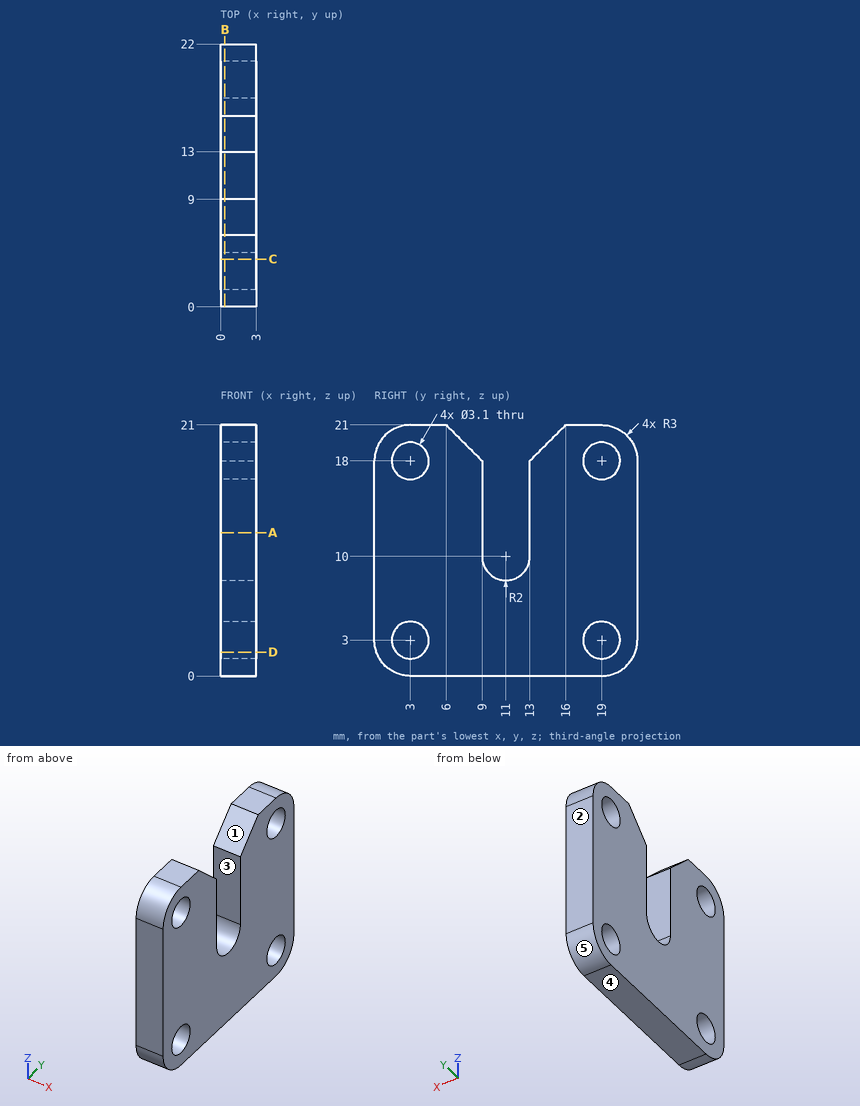
Here's the drawing with two shaded views (mm, measured from the low corner). I have some questions. A direction names the side the tool comes from. Round coordinates to 2 decimals unless told otherwise and drop trailing zeros. Loops run counter-clockwise (first coordinate to the right, second up) from the corner with the lowest first, then second, coordinate; pieces in that order, holes last.
Item 1: Suppose I cut it at B-B, the plane x = 0.35. Write out the boundary of the cut face in (y, z), then the cut area to 3 significant figures.
Item 2: Please list where these lines run through material, in increasing order: L1, parallel to Y at x = 2.1, z = 3; L2, parallel to Y at x = 0.95, z = 12.25; L3, parallel to Y at x = 1, z = 17.25.
Item 3: Will these pins go through, and if not, where does the flat tip stop? pin 1 Ø1.5 at (x, z) = (1, 14.5) entering from -Y; pin 2 Ø3 at (y, z) = (19, 18) entering from +X.
Item 4: Suppose I cut it at C-C, the plane y = 4. Write out the boundary of the cut face in (x, z), then the cut area to 3 significant figures.
Item 5: Suppose I cut it at D-D, the plane z = 2. Write out the boundary of the cut face in (x, y).
Item 6: Which directions (+Z, -Z, +X, -X, +Y, -Y) give clear straight access to the entire face, cutting with the end or side of a thin tool? Please do the marked faces 1 and 2.
Item 7: Suppose I cut it at A-A, the plane z = 12. Write out the boundary of the cut face in (x, y).
Item 8: If we mould it in two halves opening along Y, with no side actions, what happens to the marked faces 3, 4 and 5? For each: +Y half, -Y half, draft (parallel to the pull), parting line (faces both ways), or undercut.
Reported:
1. outline: (0, 3) arc R3 ccw to (3, 0) - (19, 0) arc R3 ccw to (22, 3) - (22, 18) arc R3 ccw to (19, 21) - (16, 21) - (13, 18) - (13, 10) arc R2 cw to (9, 10) - (9, 18) - (6, 21) - (3, 21) arc R3 ccw to (0, 18) - close; hole circle Ø3.1 at (3, 3); hole circle Ø3.1 at (3, 18); hole circle Ø3.1 at (19, 3); hole circle Ø3.1 at (19, 18)
1. area: 365 mm2
2. L1: y = 0 to 1.45, 4.55 to 17.45, 20.55 to 22
2. L2: y = 0 to 9, 13 to 22
2. L3: y = 0 to 1.64, 4.36 to 9, 13 to 17.64, 20.36 to 22
3. pin 1: stops at y = 0
3. pin 2: passes through
4. outline: (0, 0) - (3, 0) - (3, 1.82) - (0, 1.82) - close; (0, 4.18) - (3, 4.18) - (3, 16.82) - (0, 16.82) - close; (0, 19.18) - (3, 19.18) - (3, 21) - (0, 21) - close
4. area: 48.8 mm2
5. outline: (0, 0.17) - (3, 0.17) - (3, 1.82) - (0, 1.82) - close; (0, 4.18) - (3, 4.18) - (3, 17.82) - (0, 17.82) - close; (0, 20.18) - (3, 20.18) - (3, 21.83) - (0, 21.83) - close
6. face 1: +Z, +X, -X
6. face 2: +Z, -Z, +X, -X, +Y
7. outline: (0, 0) - (3, 0) - (3, 9) - (0, 9) - close; (0, 13) - (3, 13) - (3, 22) - (0, 22) - close
8. face 3: undercut
8. face 4: draft
8. face 5: +Y half
